CAD build for the part. Positions are in the model's coordinates, mm. A direction names the side the tool comes from. Coordinates: 2 decimals unless noted, no trailing zeros. Order: outer loops, then holes, each group sorted by start corner. A loop starts at its lowest first (then second) coordinate and runs counter-clockwise, first axis right, second up.
from build123d import *

# Parameters (mm, degrees)
CYLINDER028_R          = 1.4
CYLINDER028_DEPTH      = 19
CYLINDER028_ROLL_ANGLE = 90
CYLINDER031_R          = 1.4
CYLINDER031_DEPTH      = 19
CYLINDER031_ROLL_ANGLE = 90
CYLINDER032_R          = 1.4
CYLINDER032_DEPTH      = 19
CYLINDER032_ROLL_ANGLE = 90
CYLINDER027_R          = 1.4
CYLINDER027_DEPTH      = 19
CYLINDER027_ROLL_ANGLE = 90
CYLINDER021_R          = 1
CYLINDER021_DEPTH      = 30
CYLINDER022_R          = 1
CYLINDER022_DEPTH      = 30
BOX001007_W            = 4
BOX001007_H            = 4.2
BOX001007_DEPTH        = 27
CYLINDER020_R          = 2.1
CYLINDER020_DEPTH      = 30
CYLINDER023_R          = 2.1
CYLINDER023_DEPTH      = 30
CYLINDER024_R          = 1
CYLINDER024_DEPTH      = 30
BOX001008_W            = 4
BOX001008_H            = 2
BOX001008_DEPTH        = 27
CYLINDER025_R          = 1
CYLINDER025_DEPTH      = 30
BOX001009_W            = 4
BOX001009_H            = 2
BOX001009_DEPTH        = 27
CYLINDER016_R          = 3.5
CYLINDER016_DEPTH      = 30
CYLINDER017_R          = 4.7
CYLINDER017_DEPTH      = 30
CYLINDER018_R          = 10
CYLINDER018_DEPTH      = 30
CYLINDER026_R          = 10
CYLINDER026_DEPTH      = 30
CYLINDER019_R          = 10
CYLINDER019_DEPTH      = 30
BOX001006_W            = 39
BOX001006_H            = 24
BOX001006_DEPTH        = 10
CHAMFER_SIZE           = 1
CHAMFER014_SIZE        = 0.5


with BuildPart() as cylinder028:
    # Cylinder028 → Cylinder028 (new body)
    with BuildSketch(Plane.XY):
        Circle(CYLINDER028_R)
    extrude(amount=CYLINDER028_DEPTH)


with BuildPart() as cylinder028_1:
    # Cylinder028 roll: moved
    add(cylinder028.part.rotate(Axis((0, 0, 0), (1, 0, 0)), CYLINDER028_ROLL_ANGLE))


with BuildPart() as cylinder028_2:
    # Cylinder028 placement: moved
    add(cylinder028_1.part.moved(Location((4, 24, 6))))


with BuildPart() as cylinder031:
    # Cylinder031 → Cylinder031 (new body)
    with BuildSketch(Plane.XY):
        Circle(CYLINDER031_R)
    extrude(amount=CYLINDER031_DEPTH)


with BuildPart() as cylinder031_1:
    # Cylinder031 roll: moved
    add(cylinder031.part.rotate(Axis((0, 0, 0), (1, 0, 0)), CYLINDER031_ROLL_ANGLE))


with BuildPart() as cylinder031_2:
    # Cylinder031 placement: moved
    add(cylinder031_1.part.moved(Location((-4, 24, 6))))


with BuildPart() as part_mirroring:
    # Part__Mirroring: instance of Cylinder031
    add(cylinder031_2.part.mirror(Plane(origin=(0, 0, 0), x_dir=(1, 0, 0), z_dir=(0, 1, 0))))


with BuildPart() as cylinder032:
    # Cylinder032 → Cylinder032 (new body)
    with BuildSketch(Plane.XY):
        Circle(CYLINDER032_R)
    extrude(amount=CYLINDER032_DEPTH)


with BuildPart() as cylinder032_1:
    # Cylinder032 roll: moved
    add(cylinder032.part.rotate(Axis((0, 0, 0), (1, 0, 0)), CYLINDER032_ROLL_ANGLE))


with BuildPart() as cylinder032_2:
    # Cylinder032 placement: moved
    add(cylinder032_1.part.moved(Location((4, 24, 6))))


with BuildPart() as part_mirroring001:
    # Part__Mirroring001: instance of Cylinder032
    add(cylinder032_2.part.mirror(Plane(origin=(0, 0, 0), x_dir=(1, 0, 0), z_dir=(0, 1, 0))))


with BuildPart() as m3_tap_a:
    # Cylinder027 → Cylinder027 (new body)
    with BuildSketch(Plane.XY):
        Circle(CYLINDER027_R)
    extrude(amount=CYLINDER027_DEPTH)


with BuildPart() as m3_tap_a_1:
    # Cylinder027 roll: moved
    add(m3_tap_a.part.rotate(Axis((0, 0, 0), (1, 0, 0)), CYLINDER027_ROLL_ANGLE))


with BuildPart() as m3_tap_a_2:
    # Cylinder027 placement: moved
    add(m3_tap_a_1.part.moved(Location((-4, 24, 6))))

    # Fusion056: union Cylinder028, Part__Mirroring, Part__Mirroring001
    add(cylinder028_2.part)
    add(part_mirroring.part)
    add(part_mirroring001.part)


with BuildPart() as cylinder021:
    # Cylinder021 → Cylinder021 (new body)
    with BuildSketch(Plane(origin=(17, -4.5, -12.5), x_dir=(1, 0, 0), z_dir=(0, 0, 1))):
        Circle(CYLINDER021_R)
    extrude(amount=CYLINDER021_DEPTH)


with BuildPart() as cylinder022:
    # Cylinder022 → Cylinder022 (new body)
    with BuildSketch(Plane(origin=(17, 4.5, -12.5), x_dir=(1, 0, 0), z_dir=(0, 0, 1))):
        Circle(CYLINDER022_R)
    extrude(amount=CYLINDER022_DEPTH)


with BuildPart() as cube005:
    # Box001007 → Box001007 (new body)
    with BuildSketch(Plane(origin=(13, -2.1, -11), x_dir=(1, 0, 0), z_dir=(0, 0, 1))):
        with Locations((2, 2.1)):
            Rectangle(BOX001007_W, BOX001007_H)
    extrude(amount=BOX001007_DEPTH)


with BuildPart() as cylinder020:
    # Cylinder020 → Cylinder020 (new body)
    with BuildSketch(Plane(origin=(17, 0, -12.5), x_dir=(1, 0, 0), z_dir=(0, 0, 1))):
        Circle(CYLINDER020_R)
    extrude(amount=CYLINDER020_DEPTH)


with BuildPart() as cylinder023:
    # Cylinder023 → Cylinder023 (new body)
    with BuildSketch(Plane(origin=(13, 0, -12.5), x_dir=(1, 0, 0), z_dir=(0, 0, 1))):
        Circle(CYLINDER023_R)
    extrude(amount=CYLINDER023_DEPTH)


with BuildPart() as cylinder024:
    # Cylinder024 → Cylinder024 (new body)
    with BuildSketch(Plane(origin=(13, -4.5, -12.5), x_dir=(1, 0, 0), z_dir=(0, 0, 1))):
        Circle(CYLINDER024_R)
    extrude(amount=CYLINDER024_DEPTH)


with BuildPart() as cube006:
    # Box001008 → Box001008 (new body)
    with BuildSketch(Plane(origin=(13, -5.5, -11), x_dir=(1, 0, 0), z_dir=(0, 0, 1))):
        with Locations((2, 1)):
            Rectangle(BOX001008_W, BOX001008_H)
    extrude(amount=BOX001008_DEPTH)


with BuildPart() as cylinder025:
    # Cylinder025 → Cylinder025 (new body)
    with BuildSketch(Plane(origin=(13, 4.5, -12.5), x_dir=(1, 0, 0), z_dir=(0, 0, 1))):
        Circle(CYLINDER025_R)
    extrude(amount=CYLINDER025_DEPTH)


with BuildPart() as motor_slots:
    # Box001009 → Box001009 (new body)
    with BuildSketch(Plane(origin=(13, 3.5, -11), x_dir=(1, 0, 0), z_dir=(0, 0, 1))):
        with Locations((2, 1)):
            Rectangle(BOX001009_W, BOX001009_H)
    extrude(amount=BOX001009_DEPTH)

    # Fusion052: union Cylinder021, Cylinder022, Cube005, Cylinder020, Cylinder023, Cylinder024, Cube006, Cylinder025
    add(cylinder021.part)
    add(cylinder022.part)
    add(cube005.part)
    add(cylinder020.part)
    add(cylinder023.part)
    add(cylinder024.part)
    add(cube006.part)
    add(cylinder025.part)


with BuildPart() as cylinder016:
    # Cylinder016 → Cylinder016 (new body)
    with BuildSketch(Plane.XY.offset(-12)):
        Circle(CYLINDER016_R)
    extrude(amount=CYLINDER016_DEPTH)


with BuildPart() as cylinder017:
    # Cylinder017 → Cylinder017 (new body)
    with BuildSketch(Plane.XY.offset(-21.5)):
        Circle(CYLINDER017_R)
    extrude(amount=CYLINDER017_DEPTH)


with BuildPart() as cylinder018:
    # Cylinder018 → Cylinder018 (new body)
    with BuildSketch(Plane.XY.offset(-25.5)):
        Circle(CYLINDER018_R)
    extrude(amount=CYLINDER018_DEPTH)


with BuildPart() as cylinder026:
    # Cylinder026 → Cylinder026 (new body)
    with BuildSketch(Plane(origin=(15, 0, -25.5), x_dir=(1, 0, 0), z_dir=(0, 0, 1))):
        Circle(CYLINDER026_R)
    extrude(amount=CYLINDER026_DEPTH)


with BuildPart() as fusion054:
    # Cylinder019 → Cylinder019 (new body)
    with BuildSketch(Plane(origin=(16, 0, -25.5), x_dir=(1, 0, 0), z_dir=(0, 0, 1))):
        Circle(CYLINDER019_R)
    extrude(amount=CYLINDER019_DEPTH)

    # Fusion053: union Cylinder016, Cylinder017, Cylinder018, Cylinder026
    add(cylinder016.part)
    add(cylinder017.part)
    add(cylinder018.part)
    add(cylinder026.part)

    # Fusion054: union motor-slots
    add(motor_slots.part)


with BuildPart() as gearbox:
    # Box001006 → Box001006 (new body)
    with BuildSketch(Plane(origin=(-12, -12, 0), x_dir=(1, 0, 0), z_dir=(0, 0, 1))):
        with Locations((19.5, 12)):
            Rectangle(BOX001006_W, BOX001006_H)
    extrude(amount=BOX001006_DEPTH)

    # Cut005: cut Fusion054
    add(fusion054.part, mode=Mode.SUBTRACT)

    # Chamfer
    chamfer_edges = [gearbox.edges().sort_by_distance(p)[0] for p in [
        (12, 4.5, 4.5),
        (15, 3.5, 4.5),
        (17.707107, 3.792893, 4.5),
        (17.707107, 5.207107, 4.5),
        (15, 5.5, 4.5),
        (17.707107, -5.207107, 4.5),
        (17.707107, -3.792893, 4.5),
        (15, -3.5, 4.5),
        (12, -4.5, 4.5),
        (15, -5.5, 4.5),
    ]]
    chamfer(chamfer_edges, length=CHAMFER_SIZE)

    # Cut007: cut M3-tap-a
    add(m3_tap_a_2.part, mode=Mode.SUBTRACT)

    # Chamfer014
    chamfer014_edges = [gearbox.edges().sort_by_distance(p)[0] for p in [
        (18.484924, 1.484924, 10),
        (15, 2.1, 10),
        (10.9, 0, 10),
        (15, -2.1, 10),
        (18.484924, -1.484924, 10),
    ]]
    chamfer(chamfer014_edges, length=CHAMFER014_SIZE)


solid = gearbox.part
1) Which spindle directions (+Z, -Z, +X, -X, +Y, -Y) get a long thin tool onto all of the face, cutting with end or side? Do faces 1 (the conical face through (10.765, -0.049, 9.635)), 2 (the cylindrical face through (-2.71, -8.55, 5.46)), 3 (the cylindrical face through (18, 4.5, 7.7)), 4 (the conical face through (18.3, 4.5, 5.2)). Say none if no direction does.
2) Slice it at C-C (z = 7). Give the number of separate pieces and of enclosed holes in the cut face, plus the area to 3 significant figures.
3) Slice it at B-B (x = 0). List the corners of the cut face in (y, z), plus the area to 3 significant figures.
4) Drill centre lines: probe 1 along X at (y, z) = (0, 6.35); probe 2 along Y at (x, z) = (14.5, 9.5); probe 3 along Y at (x, z) = (0, 6.75). Where is each one in solid material? Low to high.
5) Pin check, flat tips, straight feed: P1, Ø5.5, axis at x = 0, y = 0, coming from the +Z side; P2, Ø10, axis at x = 2.5, y = 2, coming from the -Z side; P3, Ø1.7, axis at x = -4, z = 6, coming from the +Y side. Stop position of each tip, or through.
6) Slice it at A-A (y = 0). List the corners of the cut face in (x, z).
7) Two-plate mould, pull along Y, no slides. Class faces 5 (the flat face through (7, -12, 5)), 6 (the cylindrical face through (-1.02, -4.59, 6.47)), 7 (the flat face through (27, 0, 5)): released by +Y, released by -Y, zero draft, split by the parting line, or undercut.
8) Slice it at D-D (x = -7.5). List the corners of the cut face in (y, z), plus the area to 3 significant figures.
Worked out:
1. face 1: +Z
1. face 2: -Y
1. face 3: +Z, -Z
1. face 4: -Z
2. separate pieces: 1
2. enclosed holes: 4
2. area: 759 mm2
3. outline: (-12, 0) - (-10, 0) - (-10, 4.5) - (-4.7, 4.5) - (-4.7, 8.5) - (-3.5, 8.5) - (-3.5, 10) - (-12, 10) - close; (3.5, 8.5) - (4.7, 8.5) - (4.7, 4.5) - (10, 4.5) - (10, 0) - (12, 0) - (12, 10) - (3.5, 10) - close
3. area: 102 mm2
4. probe 1: x = -12 to -4.7, 4.7 to 10.9, 19.1 to 27
4. probe 2: y = -12 to -5.5, -3.5 to -2.1, 2.1 to 3.5, 5.5 to 12
4. probe 3: y = -12 to -4.7, 4.7 to 12
5. P1: passes through
5. P2: stops at z = 4.5
5. P3: stops at y = 5
6. outline: (-12, 0) - (-10, 0) - (-10, 4.5) - (-4.7, 4.5) - (-4.7, 8.5) - (-3.5, 8.5) - (-3.5, 10) - (-12, 10) - close; (3.5, 8.5) - (4.7, 8.5) - (4.7, 4.5) - (10.9, 4.5) - (10.9, 9.5) - (10.4, 10) - (3.5, 10) - close; (19.1, 4.5) - (26, 4.5) - (26, 0) - (27, 0) - (27, 10) - (19.6, 10) - (19.1, 9.5) - close
7. face 5: released by -Y
7. face 6: undercut
7. face 7: zero draft
8. outline: (-12, 0) - (-6.61, 0) - (-6.61, 4.5) - (6.61, 4.5) - (6.61, 0) - (12, 0) - (12, 10) - (-12, 10) - close
8. area: 180 mm2
